from build123d import *

# Parameters (mm, degrees)
CROQUIS1_R              = 26
SALIENTE_EXTRUIR1_DEPTH = 20
VACIADO1_T              = -3
REDONDEO1_R             = 1.5
CROQUIS2_R              = 15
SALIENTE_EXTRUIR2_DEPTH = 2
REDONDEO2_R             = 1.5
CROQUIS5_R              = 5
SALIENTE_EXTRUIR3_DEPTH = 17
CORTAR_EXTRUIR3_DEPTH   = 7
CORTAR_EXTRUIR5_DEPTH   = 10
CROQUIS12_R             = 2.975585662
CORTAR_EXTRUIR4_DEPTH   = 12


with BuildPart() as part:
    # Croquis1 → Saliente-Extruir1 (new body)
    with BuildSketch(Plane(origin=(0, 0, 0), x_dir=(1, 0, 0), z_dir=(0, 1, 0))):
        with Locations(Location((0, 0, 0), (0, 0, 270))):
            Circle(CROQUIS1_R)
    extrude(amount=SALIENTE_EXTRUIR1_DEPTH)

    # Vaciado1
    vaciado1_openings = [part.faces().sort_by_distance(p)[0] for p in [
        (0, 20, 0),
    ]]
    offset(amount=VACIADO1_T, openings=vaciado1_openings, kind=Kind.INTERSECTION)

    # Redondeo1
    redondeo1_edges = [part.edges().sort_by_distance(p)[0] for p in [
        (0, 0, -26),
    ]]
    fillet(redondeo1_edges, radius=REDONDEO1_R)

    # Croquis2 → Saliente-Extruir2 (add)
    with BuildSketch(Plane.XZ):
        with Locations(Location((0, 0, 0), (0, 0, 90))):
            Circle(CROQUIS2_R)
    extrude(amount=SALIENTE_EXTRUIR2_DEPTH)

    # Redondeo2
    redondeo2_edges = [part.edges().sort_by_distance(p)[0] for p in [
        (0, -2, -15),
    ]]
    fillet(redondeo2_edges, radius=REDONDEO2_R)

    # Croquis5 → Saliente-Extruir3 (add)
    with BuildSketch(Plane(origin=(0, 3, 0), x_dir=(1, 0, 0), z_dir=(0, 1, 0))):
        with Locations(Location((0, 0, 0), (0, 0, 270))):
            Circle(CROQUIS5_R)
    extrude(amount=SALIENTE_EXTRUIR3_DEPTH)

    # Croquis6 → Cortar-Extruir3 (cut)
    with BuildSketch(Plane(origin=(0, 20, 0), x_dir=(1, 0, 0), z_dir=(0, 1, 0))):
        with BuildLine():
            ThreePointArc((1.9, 2.05669638), (0, 2.8), (-1.9, 2.05669638))
            Line((-1.9, 2.05669638), (-1.9, -2.05669638))
            ThreePointArc((-1.9, -2.05669638), (0, -2.8), (1.9, -2.05669638))
            Line((1.9, -2.05669638), (1.9, 2.05669638))
        make_face()
    extrude(amount=-CORTAR_EXTRUIR3_DEPTH, mode=Mode.SUBTRACT)

    # Croquis10 → Refrentado para tornillo con cabeza troncocónica de M2.51 (revolve, cut)
    with BuildSketch(Plane(origin=(0, -2, 0), x_dir=(0, 0, -1), z_dir=(1, 0, 0))):
        Polygon((0, 0), (0, 22), (1.45, 22), (1.45, 2.1), (3, 2.1), (3, 0), align=None)
    revolve(axis=Axis((0, -8.35, 0), (0, 1, 0)), mode=Mode.SUBTRACT)

    # Croquis4 → Cortar-Extruir5 (cut)
    with BuildSketch(Plane.XZ.offset(2)):
        with BuildLine():
            ThreePointArc((-5.465091238, -12.344341933), (-0.32920888, -13.495985385), (4.856716063, -12.59612278))
            add(Edge.make_bspline(
                [(4.856716063, -12.59612278), (0.260062293, 4.863404328), (-5.465091238, -12.344341933)],
                knots=[0.092611361, 0.092611361, 0.092611361, 0.907859472, 0.907859472, 0.907859472], degree=2))
        make_face()
        with BuildLine():
            add(Edge.make_bspline(
                [(-12.59612278, -4.856716063), (4.863404328, -0.260062293), (-12.344341933, 5.465091238)],
                knots=[0.092611361, 0.092611361, 0.092611361, 0.907859472, 0.907859472, 0.907859472], degree=2))
            ThreePointArc((-12.344341933, 5.465091238), (-13.495985385, 0.32920888), (-12.59612278, -4.856716063))
        make_face()
        with BuildLine():
            add(Edge.make_bspline(
                [(-4.564383108, 12.704975673), (-0.276925472, -4.973532137), (5.206643951, 12.455555338)],
                knots=[0.037040057, 0.037040057, 0.037040057, 0.963168016, 0.963168016, 0.963168016], degree=2))
            ThreePointArc((5.206643951, 12.455555338), (0.344495825, 13.495603826), (-4.564383108, 12.704975673))
        make_face()
        with BuildLine():
            ThreePointArc((13.5, 0), (13.272107171, 2.470054906), (12.59612278, 4.856716063))
            add(Edge.make_bspline(
                [(12.59612278, 4.856716063), (-4.863404328, 0.260062293), (12.344341933, -5.465091238)],
                knots=[0.092611361, 0.092611361, 0.092611361, 0.907859472, 0.907859472, 0.907859472], degree=2))
            ThreePointArc((12.344341933, -5.465091238), (13.207925956, -2.792971885), (13.5, 0))
        make_face()
    extrude(amount=-CORTAR_EXTRUIR5_DEPTH, mode=Mode.SUBTRACT)

    # Croquis12 → Cortar-Extruir4 (cut)
    with BuildSketch(Plane.XZ.offset(-0.1)):
        with Locations(Location((0, 0, 0), (0, 0, 270))):
            Circle(CROQUIS12_R)
    extrude(amount=-CORTAR_EXTRUIR4_DEPTH, mode=Mode.SUBTRACT)


solid = part.part
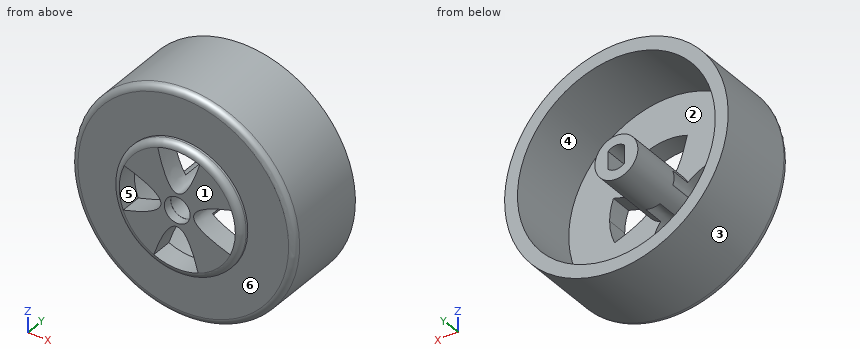
For this review, take the finished solid that the model builds, in its own axes (mm). Face numbers are marked on the shaded views. A direction names the side the tool comes from. Round coordinates to 2 decimals unless told otherwise and drop trailing zeros. Order: outer loops, then holes, each group sorted by start corner. A loop starts at its lowest first (then second) coordinate and runs counter-clockwise, first axis right, second up. Notation, with made-up numbers: M -12,37.25 L 4,37.25 A19 ccw 4,54.25 Z; hole C 65.5,35 d7. An arc over 180 degrees is marked long. Write each question's results on one line, items separated by ' | '. Start each with the question number.
1. Add section A-A (y = 15.75). State the section outline as (x, z) points, then the cut area to 3 significant figures.
2. Tool access review of the marked faces 4, 5 and 6: name each direction out of +Z, -Z, +X, -X, +Y, -Y from which nothing blocks a thin tool from reaching the whole face with its end or side.
3. Clearance check with flat-ended pins moving along their axes: pin 1 Ø0.6 at (x, z) = (0, -4.5) entering from -Y; pin 2 Ø4 at (x, z) = (1.5, -14.5) entering from +Y; pin 3 Ø6 at (x, y) = (-9.5, 3.5) entering from -Z. State where each tip first meets the part, or that it passes through.
4. Add section B-B (x = 0). State how many separate pieces and enclosed holes the cut face has, then the cut area to 3 significant figures.
5. Draft analysis for pull direction X (two halves, no side actions). For the marked faces 1, 2 and 3, state which applies: pulls with the +X half, pulls with the -X half, needs draft (parallel to the pull), parting line crosses it, or undercut.
6. To check wall thickness, follow L1, parallel to X at y = 8.25, z = 0; L2, parallel to X at y = 13.5, z = 0; L3, parallel to Z at x = -4.5, y = 12.5. State the ranges of each line that lie inside material, in increasing order. Write a range as [from, to].
Output values:
1) outline: C 0,0 d52; C 0,0 d10; hole C 0,0 d46; hole M -1.9,-2.06 A2.8 ccw 1.9,-2.06 L 1.9,2.06 A2.8 ccw -1.9,2.06 Z | area: 521 mm^2
2) face 4: +Y | face 5: +Y, -Y | face 6: -Y
3) pin 1: y = 8 | pin 2: y = 3 | pin 3: z = -25.17
4) separate pieces: 4 | enclosed holes: 0 | area: 251 mm^2
5) face 1: needs draft | face 2: undercut | face 3: parting line crosses it
6) L1: [-26, -23], [-5, -2.98], [2.98, 5], [23, 26] | L2: [-26, -23], [-5, -1.9], [1.9, 5], [23, 26] | L3: [-25.61, -22.56], [-2.18, 2.18], [22.56, 25.61]
